```python
from build123d import *

# Parameters (mm, degrees)
EXTRUDE_1_DEPTH = 650


with BuildPart() as part:
    # 草图5 → 凸台-拉伸1 (new body, symmetric)
    with BuildSketch(Plane(origin=(0, 0, 0), x_dir=(1, 0, 0), z_dir=(0, 1, 0))):
        with BuildLine():
            Line((-267.514659832, 138.60716948), (-385, 4.891224703))
            Line((-385, 4.891224703), (-385, -4.891224703))
            Line((-385, -4.891224703), (-267.514659832, -138.60716948))
            ThreePointArc((-267.514659832, -138.60716948), (-259.47883349, -149.810174364), (-253.794659832, -162.37090656))
            Line((-253.794659832, -162.37090656), (-196.735924848, -330.974168106))
            Line((-196.735924848, -330.974168106), (-188.264075152, -335.865392808))
            Line((-188.264075152, -335.865392808), (-13.72, -300.978076039))
            ThreePointArc((-13.72, -300.978076039), (0, -299.620348729), (13.72, -300.978076039))
            Line((13.72, -300.978076039), (188.264075152, -335.865392808))
            Line((188.264075152, -335.865392808), (196.735924848, -330.974168106))
            Line((196.735924848, -330.974168106), (253.794659832, -162.37090656))
            ThreePointArc((253.794659832, -162.37090656), (259.47883349, -149.810174364), (267.514659832, -138.60716948))
            Line((267.514659832, -138.60716948), (385, -4.891224703))
            Line((385, -4.891224703), (385, 4.891224703))
            Line((385, 4.891224703), (267.514659832, 138.60716948))
            ThreePointArc((267.514659832, 138.60716948), (259.47883349, 149.810174364), (253.794659832, 162.37090656))
            Line((253.794659832, 162.37090656), (196.735924848, 330.974168106))
            Line((196.735924848, 330.974168106), (188.264075152, 335.865392808))
            Line((188.264075152, 335.865392808), (13.72, 300.978076039))
            ThreePointArc((13.72, 300.978076039), (0, 299.620348729), (-13.72, 300.978076039))
            Line((-13.72, 300.978076039), (-188.264075152, 335.865392808))
            Line((-188.264075152, 335.865392808), (-196.735924848, 330.974168106))
            Line((-196.735924848, 330.974168106), (-253.794659832, 162.37090656))
            ThreePointArc((-253.794659832, 162.37090656), (-259.47883349, 149.810174364), (-267.514659832, 138.60716948))
        make_face()
    extrude(amount=EXTRUDE_1_DEPTH, both=True)


solid = part.part
```
Check sheet for the modelled part. Datum: model origin and axes. Units: mm. A direction names the side the tool comes from. Coordinates: 2 decimals unless noted, no trailing zeros. Write each loop counter-clockwise with the first axis right and the second up, starting at its lowest first coordinate (ties: lowest second). Pieces come first, ordered by that corner, then holes. Notation, with made-up numbers: M -9.75,67.25 L 31.25,67.25 A7 ccw 31.25,74.25 Z; hole C 69.5,53 d1. An arc over 180 degrees is marked long. Use one line per item in the form item = value.
Item 1: Gauge pin test, flat ends, axial feed: pin 1 Ø1 at (y, z) = (244.5, -101.5) entering from +X; pin 2 Ø1.5 at (y, z) = (242, 191.5) entering from -X; pin 3 Ø2 at (x, y) = (43, 394) entering from -Z. Record the tip position at first contact, or that the pin passes through.
Answer below:
pin_1 = 300.56
pin_2 = -244.19
pin_3 = -307.03
Item 2: Sectioned sample at C-C, the plane x = -60. Record the cut outline in (y, z), and give its area (3 significant figures).
Answer below:
outline = M -650,-310.23 L 650,-310.23 L 650,310.23 L -650,310.23 Z
area = 807,000 mm^2
Item 3: Sectioned sample at B-B, the plane z = 232.5. Record the cut outline in (x, y), and give its area (3 significant figures).
Answer below:
outline = M -230.06,-650 L 230.06,-650 L 230.06,650 L -230.06,650 Z
area = 598,000 mm^2
Item 4: Material ranges on L1, parallel to X at y = 44, z = -187; L2, parallel to Z at x = 196.5, y = -109.5; L3, parallel to Z at x = -92.5, y = 183, recorded low to high. Write a range as from..to.
Answer below:
L1 = -245.46..245.46
L2 = -331.11..331.11
L3 = -316.72..316.72
Item 5: Release check for a two-part mould opening along X. For faces 4 (the face through (102.214, 9.1, -318.666)), 5 (the face through (-225.665, 9.1, 245.492)), 6 (the face through (-5, 650, -5)) record: pulls with the +X half, pulls with the -X half, needs draft (parallel to the pull), parting line crosses it, or undercut.
Answer below:
face_4 = undercut
face_5 = pulls with the -X half
face_6 = needs draft
Item 6: Set-up check for faces 1 (the face through (99.77, 9.1, 318.178)), 2 (the face through (327.08, 9.1, -70.81)), 3 (the face through (-99.77, 9.1, -318.178)): record each of +Z, -Z, +X, -X, +Y, -Y from which the full face is reachable in a straight line by a thin tool's end or side.
Answer below:
face_1 = +Z, +Y, -Y
face_2 = -Z, +X, +Y, -Y
face_3 = -Z, +Y, -Y
Item 7: Sectioned sample at A-A, the plane y = -279. Record the cut outline in (x, z), and give its area (3 significant figures).
Answer below:
outline = M -385,-4.89 L -267.51,-138.61 A70 cw -253.79,-162.37 L -196.74,-330.97 L -188.26,-335.87 L -13.72,-300.98 A70 cw 13.72,-300.98 L 188.26,-335.87 L 196.74,-330.97 L 253.79,-162.37 A70 cw 267.51,-138.61 L 385,-4.89 L 385,4.89 L 267.51,138.61 A70 cw 253.79,162.37 L 196.74,330.97 L 188.26,335.87 L 13.72,300.98 A70 cw -13.72,300.98 L -188.26,335.87 L -196.74,330.97 L -253.79,162.37 A70 cw -267.51,138.61 L -385,4.89 Z
area = 348,000 mm^2
